Work out the finished part from the listing and answer in its coordinate system (mm). Face numbers are marked on the shaded views. A direction names the side the tool comes from. Round coordinates to 2 decimals unless told otherwise and drop trailing zeros. Order: outer loops, then holes, each group sorted by start corner. A loop starts at its lowest first (then second) coordinate and runs counter-clockwise, first axis right, second up. Notation, with made-up numbers: (-20, 7) - (-6, 7) arc R6 ccw to (-6, 18) - close; hole circle Ø2 at (-22, 50.5). An arc over 180 degrees is marked (long way). Use one line per item in the form item = value. Start each with the question number.
Q1. For a pull along X with two mould halves and no side action, classify the marked faces 3, 4, 5 and 6 as +X half, -X half, draft (parallel to the pull), parting line (faces both ways), or undercut.
Q2. Given P1, Ø7, axis at x = -125.15, y = 32, coming from the -Z side; P2, Ø10, axis at x = 105, z = -31.5, coming from the -Y side; P3, Ø5, axis at x = 199.5, z = -74.35, coming from the +Y side, each flat-ended and moving along its own axis, determine where each tip first touches the part or whether it passes through.
Q3. The part is cut by section A-A on z = -26. Determine the outline of the cut face in (x, y), plus the area to 3 significant figures.
Q4. The part is cut by section B-B on z = 50.5. Determine the outline of the cut face in (x, y).
Q5. Which of the six approach directions +Z, -Z, +X, -X, +Y, -Y give full straight-line access (tool end or side, diameter ignored) to the marked faces 1 and 2?
Q6. The part is cut by section C-C on x = 67. Determine the outline of the cut face in (y, z), plus the area to 3 significant figures.
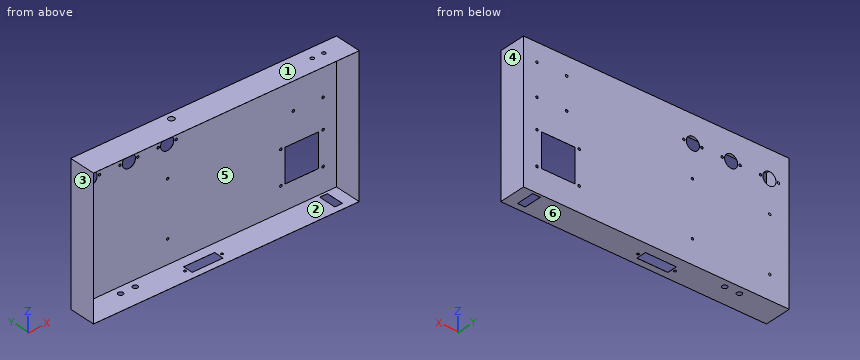
Autodesk Inventor part; units mm, degrees
ref_plane "YZ Plane" through (0, 0, 0) normal (1, 0, 0) x (0, 1, 0)
ref_plane "XZ Plane" through (0, 0, 0) normal (0, 1, 0) x (-1, 0, 0)
ref_plane "XY Plane" through (0, 0, 0) normal (0, 0, 1) x (1, 0, 0)
sketch "Sketch1" plane through (0, 0, 0) normal (0, 1, 0) x (-1, 0, 0)
  line L0 (222, -115) -> (-222, -115)
  line L1 (-222, -115) -> (-222, 115)
  line L2 (-222, 115) -> (222, 115)
  line L3 (222, 115) -> (222, -115)
  line L4 (0, -161) -> (0, 161)
  line L5 (310.8, 0) -> (-310.8, 0)
  point P0 (0, 0)
  dimension "d0" = 444
  dimension "d1" = 230
extrude "Extrusion1" add sketch "Sketch1" along normal blind 45
sketch "Sketch10" plane through (0, 0, 0) normal (0, -1, 0) x (1, 0, 0)
  line L0 (-221.88, 114.88) -> (221.88, 114.88)
  line L1 (221.88, 114.88) -> (221.88, -114.88)
  line L2 (221.88, -114.88) -> (-221.88, -114.88)
  line L3 (-221.88, -114.88) -> (-221.88, 114.88)
  line L4 (0, -161) -> (0, 161)
  line L5 (-310.8, 0) -> (310.8, 0)
  line L6 (-222, 115) -> (-222, -115)
  line L7 (222, 115) -> (-222, 115)
  point P0 (0, 0)
  dimension "d19" = 0.12
  dimension "d20" = 0.12
extrude "Extrusion6" cut sketch "Sketch10" against normal blind 44.88 contours L0 L4 L5 L3 | L0 L1 L5 L4 | L5 L4 L2 L3 | L5 L1 L2 L4
sketch "Sketch11" plane through (0, 45, 0) normal (0, 1, 0) x (1, 0, 0)
  circle A0 centre (-189, -70) radius 11
  line L0 (-222, 115) -> (-222, -115)
  line L1 (-222, -115) -> (222, -115)
  circle A1 centre (-125, -70) radius 11
  circle A2 centre (-61, -70) radius 11
  line L2 (-221.88, 114.88) -> (-221.88, -114.88)
  line L3 (-221.88, -70) -> (1.88, -70) construction
  circle A3 centre (-174, -70) radius 2
  circle A4 centre (-204, -70) radius 2
  circle A5 centre (-140, -70) radius 2
  circle A6 centre (-110, -70) radius 2
  circle A7 centre (-76, -70) radius 2
  circle A8 centre (-46, -70) radius 2
  line L4 (-60.23, 75.55) -> (-189.48, 75.55) construction
  line L5 (-189.48, 75.55) -> (-189.48, -16.15) construction
  line L6 (-189.48, -16.15) -> (-60.23, -16.15) construction
  line L7 (-60.23, -16.15) -> (-60.23, 75.55) construction
  line L8 (222, 115) -> (-222, 115)
  circle A9 centre (-189.48, 75.55) radius 2
  circle A10 centre (-60.23, 75.55) radius 2
  circle A11 centre (-60.23, -16.15) radius 2
  circle A12 centre (-189.48, -16.15) radius 2
  point P0 (0, 0)
  dimension "d24" = 22
  dimension "d25" = 33
  dimension "d27" = 22
  dimension "d30" = 64
  dimension "d31" = 22
  dimension "d33" = 64
  dimension "d35" = 45
  dimension "d36" = 4
  dimension "d37" = 15
  dimension "d38" = 4
  dimension "d39" = 15
  dimension "d40" = 4
  dimension "d41" = 4
  dimension "d42" = 4
  dimension "d43" = 4
  dimension "d44" = 15
  dimension "d45" = 15
  dimension "d46" = 15
  dimension "d47" = 15
  dimension "d50" = 129.25
  dimension "d52" = 39.45
  dimension "d54" = 32.4
  dimension "d55" = 91.7
  dimension "d56" = 4
  dimension "d57" = 4
  dimension "d58" = 4
  dimension "d59" = 4
extrude "Extrusion7" cut sketch "Sketch11" against normal up to next
sketch "Sketch12" plane through (0, 45, 0) normal (0, 1, 0) x (1, 0, 0)
  line L0 (129, 74.35) -> (199.5, 74.35) construction
  line L1 (199.5, 74.35) -> (199.5, 18.35) construction
  line L2 (199.5, 18.35) -> (129, 18.35) construction
  line L3 (129, 18.35) -> (129, 74.35) construction
  line L4 (222, 115) -> (-222, 115)
  line L5 (199.5, 115) -> (199.5, -115) construction
  line L6 (-222, -115) -> (222, -115)
  line L7 (222, -115) -> (222, 115)
  circle A0 centre (129, 74.35) radius 2.1
  circle A1 centre (199.5, 74.35) radius 2.1
  circle A2 centre (199.5, 18.35) radius 2.1
  circle A3 centre (129, 18.35) radius 2.1
  point P0 (0, 0)
  dimension "d65" = 22.5
  dimension "d66" = 40.65
  dimension "d67" = 56
  dimension "d68" = 4.2
  dimension "d69" = 4.2
  dimension "d70" = 4.2
  dimension "d71" = 4.2
  dimension "d72" = 70.5
extrude "Extrusion8" cut sketch "Sketch12" against normal up to next
sketch "Sketch13" plane through (0, 45, 0) normal (0, 1, 0) x (1, 0, 0)
  line L0 (149.8, -31.1) -> (199.5, -31.1) construction
  line L1 (199.5, -31.1) -> (199.5, -84.5) construction
  line L2 (199.5, -84.5) -> (149.8, -84.5) construction
  line L3 (149.8, -84.5) -> (149.8, -31.1) construction
  line L4 (222, -115) -> (222, 115)
  line L5 (-222, -115) -> (222, -115)
  line L6 (199.5, 74.35) -> (199.5, 18.35) construction
  line L7 (199.5, 115) -> (199.5, -115) construction
  circle A0 centre (199.5, -31.1) radius 2.1
  circle A1 centre (149.8, -31.1) radius 2.1
  circle A2 centre (149.8, -84.5) radius 2.1
  circle A3 centre (199.5, -84.5) radius 2.1
  point P0 (0, 0)
  dimension "d75" = 49.7
  dimension "d77" = 53.4
  dimension "d79" = 30.5
  dimension "d80" = 4.2
  dimension "d81" = 4.2
  dimension "d82" = 4.2
  dimension "d83" = 4.2
extrude "Extrusion9" cut sketch "Sketch13" against normal up to next
sketch "Sketch14" plane through (0, 45, 0) normal (0, 1, 0) x (1, 0, 0)
  line L0 (199.5, 74.35) -> (199.5, 18.35) construction
  line L1 (129, 74.35) -> (199.5, 74.35) construction
  line L2 (199.5, 18.35) -> (129, 18.35) construction
  line L3 (129, 18.35) -> (129, 74.35) construction
  line L4 (135.6, 74.35) -> (191.6, 74.35)
  line L5 (191.6, 74.35) -> (191.6, 18.35)
  line L6 (191.6, 18.35) -> (135.6, 18.35)
  line L7 (135.6, 18.35) -> (135.6, 74.35)
  line L8 (121.9, 81.45) -> (206.6, 81.45) construction
  line L9 (206.6, 81.45) -> (206.6, 11.25) construction
  line L10 (206.6, 11.25) -> (121.9, 11.25) construction
  line L11 (121.9, 11.25) -> (121.9, 81.45) construction
  point P0 (0, 0)
  dimension "d86" = 56
  dimension "d87" = 56
  dimension "d88" = 7.1
  dimension "d89" = 7.1
  dimension "d90" = 7.1
  dimension "d92" = 15
  dimension "d94" = 7.1
extrude "Extrusion10" cut sketch "Sketch14" against normal up to next
sketch "Sketch16" plane through (-222, 0, 115) normal (0, 0, 1) x (1, 0, 0)
  circle A0 centre (406, 25) radius 3
  line L0 (444, 0) -> (444, 45)
  line L1 (444, 0) -> (0, 0)
  circle A1 centre (386.6, 25) radius 3
  line L2 (443.88, 0) -> (443.88, 44.88)
  line L3 (443.88, 25) -> (334.929, 25) construction
  point P0 (222, 0)
  dimension "d97" = 6
  dimension "d98" = 38
  dimension "d100" = 6
  dimension "d101" = 108.951
  dimension "d102" = 25
  dimension "d103" = 19.4
extrude "Extrusion11" cut sketch "Sketch16" against normal up to surface (0.12 mm away)
sketch "Sketch17" plane through (-222, 0, 115) normal (0, 0, 1) x (1, 0, 0)
  circle A0 centre (158, 33) radius 5
  line L0 (0, 0) -> (0, 45)
  line L1 (444, 0) -> (0, 0)
  point P0 (222, 0)
  dimension "d106" = 10
  dimension "d107" = 158
  dimension "d108" = 33
extrude "Extrusion12" cut sketch "Sketch17" against normal up to surface (0.12 mm away)
sketch "Sketch18" plane through (222, 0, -115) normal (0, 0, -1) x (-1, 0, 0)
  line L0 (19, 40.5) -> (32, 40.5)
  line L1 (32, 40.5) -> (32, 10.5)
  line L2 (32, 10.5) -> (19, 10.5)
  line L3 (19, 10.5) -> (19, 40.5)
  line L4 (19, 40.5) -> (32, 10.5) construction
  line L5 (32, 40.5) -> (19, 10.5) construction
  line L6 (0, 45) -> (444, 45)
  line L7 (0, 0) -> (0, 45)
  point P0 (222, 0)
  point P1 (25.5, 25.5)
  dimension "d111" = 13
  dimension "d112" = 30
  dimension "d113" = 4.5
  dimension "d114" = 19
extrude "Extrusion13" cut sketch "Sketch18" against normal up to surface (0.12 mm away)
sketch "Sketch19" plane through (222, 0, -115) normal (0, 0, -1) x (-1, 0, 0)
  circle A0 centre (371.75, 32) radius 4.25
  line L0 (444, 0) -> (444, 45)
  line L1 (444, 32) -> (305.1223, 32) construction
  line L2 (444, 0) -> (0, 0)
  circle A1 centre (347.15, 32) radius 4.25
  line L3 (0, 45) -> (444, 45)
  point P0 (222, 0)
  dimension "d117" = 8.5
  dimension "d118" = 138.8777
  dimension "d120" = 72.25
  dimension "d121" = 8.5
  dimension "d122" = 24.6
  dimension "d123" = 13
extrude "Extrusion14" cut sketch "Sketch19" against normal up to surface (0.12 mm away)
sketch "Sketch20" plane through (222, 0, -115) normal (0, 0, -1) x (-1, 0, 0)
  line L0 (218, 28) -> (270, 28)
  line L1 (270, 28) -> (270, 11)
  line L2 (270, 11) -> (218, 11)
  line L3 (218, 11) -> (218, 28)
  line L4 (218, 28) -> (270, 11) construction
  line L5 (270, 28) -> (218, 11) construction
  line L6 (0, 45) -> (444, 45)
  line L7 (182.7735, 19.5) -> (305.684, 19.5) construction
  line L8 (444, 0) -> (444, 45)
  circle A0 centre (213, 19.5) radius 2
  circle A1 centre (275, 19.5) radius 2
  line L9 (244, 36.5338) -> (244, 7.8411) construction
  point P0 (222, 0)
  point P1 (244, 19.5)
  point P2 (244, 19.5)
  point P3 (244, 19.5)
  dimension "d126" = 52
  dimension "d127" = 17
  dimension "d129" = 17
  dimension "d130" = 200
  dimension "d131" = 4
  dimension "d132" = 4
  dimension "d133" = 5
extrude "Extrusion15" cut sketch "Sketch20" against normal up to surface (0.12 mm away)
equation "\"d60\" = d56"
equation "\"d95\" = d56"
properties part number "Gehaeuse_Deckel"
Found:
q1.face_3 = -X half
q1.face_4 = +X half
q1.face_5 = undercut
q1.face_6 = draft
q2.P1 = 114.88
q2.P2 = 44.88
q2.P3 = 45
q3.outline = (-222, 0) - (-221.88, 0) - (-221.88, 44.88) - (135.6, 44.88) - (135.6, 45) - (-222, 45) - close; (191.6, 44.88) - (221.88, 44.88) - (221.88, 0) - (222, 0) - (222, 45) - (191.6, 45) - close
q3.area = 57.3 mm²
q4.outline = (-222, 0) - (-221.88, 0) - (-221.88, 44.88) - (221.88, 44.88) - (221.88, 0) - (222, 0) - (222, 45) - (-222, 45) - close
q5.face_1 = +Z, +X, -X, +Y, -Y
q5.face_2 = -Y
q6.outline = (0, -115) - (45, -115) - (45, 115) - (0, 115) - (0, 114.88) - (44.88, 114.88) - (44.88, -114.88) - (0, -114.88) - close
q6.area = 38.4 mm²
